The listing builds one solid part. Answer for the finished solid, in the listing's coordinates (mm). A direction names the side the tool comes from. Round coordinates to 2 decimals unless told otherwise and drop trailing zeros. Loops run counter-clockwise (first coordinate to the right, second up) from the corner with the lowest first, then second, coordinate; pieces in that order, holes last. Notation, with made-up numbers: (79, 3.25) - (85, 3.25) arc R17 cw to (85, 35.25) - close; hole circle Ø11 at (-14, -18.5). An arc over 180 degrees is marked (long way). Write item = value, one per line. Start each with the question number.
1) Straight lines are drawn through the part: line 1 along Y through (x, z) = (29, 17.5); line 2 along X through (y, z) = (10.5, 11); line 3 along X through (y, z) = (4.25, 4.25). For each, find the intervals that lie inside material, in ascending order.
2) Section B-B, the plane z = 11 is taken. Determine the outline of the cut face in (x, y), and give its area (3 significant figures).
3) Section C-C, the plane x = 29 is taken. Determine the outline of the cut face in (y, z), and give its area (3 significant figures).
4) Section A-A, the plane y = 6 is taken. Determine the outline of the cut face in (x, z), and give its area (3 significant figures).
5) A tool of negligible diameter and unlimited length cuts with its end or side. For faces 4 (the flat face through (33, 15, 9)), 5 (the flat face through (1, 15, 9)), 6 (the cylindrical face through (3, 24, 13)), 7 (the flat face through (17, 15, 21.5)), from which of +Z, -Z, +X, -X, +Y, -Y can it reach the whole face along a straight path? Write none if from no direction.
6) For a pull along Z with two mould halves and no side action, classify faces 1 (the flat face through (14, 2, 8)), 2 (the flat face through (5, 15, 22)), 3 (the flat face through (29, 15, 4)) as released by +Z, released by -Z, zero draft, split by the parting line, or undercut.
7) Section D-D, the plane y = 3 is taken. Determine the outline of the cut face in (x, z).
8) Given pin 1 Ø4 at (x, y) = (28.5, 19) entering from -Z; pin 2 Ø5 at (y, z) = (13, 7.5) entering from -X; pin 3 Ø2 at (x, z) = (11.5, 12) entering from +Y; pin 4 Ø5 at (x, z) = (17, 11) entering from -Y, each flat-ended and moving along its own axis, determine where each tip first touches the part or whether it passes through.
from build123d import *

# Parameters (mm, degrees)
CYLINDER002_R          = 7.5
CYLINDER002_DEPTH      = 4
CYLINDER002_ROLL_ANGLE = 90
BOX003_W               = 7
BOX003_H               = 34
BOX003_DEPTH           = 0.5
PAD001_DEPTH           = 27
BOX002_W               = 8
BOX002_H               = 22
BOX002_DEPTH           = 4
BOX001_W               = 1
BOX001_H               = 19
BOX001_DEPTH           = 14
PAD_DEPTH              = 31
CYLINDER001_R          = 2
CYLINDER001_DEPTH      = 30
CYLINDER_R             = 4
CYLINDER_DEPTH         = 40
CYLINDER_ROLL_ANGLE    = 90
BOX_W                  = 17
BOX_H                  = 15
BOX_DEPTH              = 22


with BuildPart() as cilindro002:
    # Cylinder002 → Cylinder002 (new body)
    with BuildSketch(Plane.XY):
        Circle(CYLINDER002_R)
    extrude(amount=CYLINDER002_DEPTH)


with BuildPart() as cilindro002_1:
    # Cylinder002 roll: moved
    add(cilindro002.part.rotate(Axis((0, 0, 0), (1, 0, 0)), CYLINDER002_ROLL_ANGLE))


with BuildPart() as cilindro002_2:
    # Cylinder002 placement: moved
    add(cilindro002_1.part.moved(Location((17, 2, 11))))


with BuildPart() as cubo003:
    # Box003 → Box003 (new body)
    with BuildSketch(Plane(origin=(10, 0, 21.5), x_dir=(1, 0, 0), z_dir=(0, 0, 1))):
        with Locations((3.5, 17)):
            Rectangle(BOX003_W, BOX003_H)
    extrude(amount=BOX003_DEPTH)


with BuildPart() as body001:
    # Sketch001 → Pad001 (new body)
    with BuildSketch(Plane.XZ):
        Polygon((0, 0), (4, 0), (0, 4), align=None)
    extrude(amount=PAD001_DEPTH)


with BuildPart() as body001_1:
    # Body001 placement: moved
    add(body001.part.moved(Location((9, 20, 0))))


with BuildPart() as cubo002:
    # Box002 → Box002 (new body)
    with BuildSketch(Plane(origin=(1, 0, 0), x_dir=(1, 0, 0), z_dir=(0, 0, 1))):
        with Locations((4, 11)):
            Rectangle(BOX002_W, BOX002_H)
    extrude(amount=BOX002_DEPTH)


with BuildPart() as cubo001:
    # Box001 → Box001 (new body)
    with BuildSketch(Plane.XY):
        with Locations((0.5, 9.5)):
            Rectangle(BOX001_W, BOX001_H)
    extrude(amount=BOX001_DEPTH)


with BuildPart() as body:
    # Sketch → Pad (new body)
    with BuildSketch(Plane.XZ):
        Polygon((0, 0), (-1, -8e-06), (-1, 1.999992), align=None)
    extrude(amount=PAD_DEPTH)


with BuildPart() as body_1:
    # Body placement: moved
    add(body.part.moved(Location((1, 18, 14))))


with BuildPart() as cilindro001:
    # Cylinder001 → Cylinder001 (new body)
    with BuildSketch(Plane(origin=(5, 6, -3), x_dir=(1, 0, 0), z_dir=(0, 0, 1))):
        Circle(CYLINDER001_R)
    extrude(amount=CYLINDER001_DEPTH)


with BuildPart() as cilindro:
    # Cylinder → Cylinder (new body)
    with BuildSketch(Plane.XY):
        Circle(CYLINDER_R)
    extrude(amount=CYLINDER_DEPTH)


with BuildPart() as cilindro_1:
    # Cylinder roll: moved
    add(cilindro.part.rotate(Axis((0, 0, 0), (1, 0, 0)), CYLINDER_ROLL_ANGLE))


with BuildPart() as cilindro_2:
    # Cylinder placement: moved
    add(cilindro_1.part.moved(Location((17, 35, 11))))


with BuildPart() as cut007:
    # Box → Box (new body)
    with BuildSketch(Plane.XY):
        with Locations((8.5, 7.5)):
            Rectangle(BOX_W, BOX_H)
    extrude(amount=BOX_DEPTH)

    # Cut: cut Cilindro
    add(cilindro_2.part, mode=Mode.SUBTRACT)

    # Cut001: cut Cilindro001
    add(cilindro001.part, mode=Mode.SUBTRACT)

    # Cut002: cut Body
    add(body_1.part, mode=Mode.SUBTRACT)

    # Cut003: cut Cubo001
    add(cubo001.part, mode=Mode.SUBTRACT)

    # Cut004: cut Cubo002
    add(cubo002.part, mode=Mode.SUBTRACT)

    # Cut005: cut Body001
    add(body001_1.part, mode=Mode.SUBTRACT)

    # Cut006: cut Cubo003
    add(cubo003.part, mode=Mode.SUBTRACT)

    # Cut007: cut Cilindro002
    add(cilindro002_2.part, mode=Mode.SUBTRACT)


with BuildPart() as fusion:
    # mirror: instance of Cut007
    add(cut007.part.mirror(Plane(origin=(17, 0, 0.020863), x_dir=(0, -1, 0), z_dir=(1, 0, 0))))

    # Fusion: union Cut007
    add(cut007.part)


with BuildPart() as mirror_of_fusion:
    # mirror001: instance of Fusion
    add(fusion.part.mirror(Plane(origin=(34, 15, 22), x_dir=(1, 0, 0), z_dir=(0, 1, 0))))


with BuildPart() as fusion001:
    # Fusion001 base: copy of Fusion
    add(fusion.part)

    # Fusion001: union Mirror of Fusion
    add(mirror_of_fusion.part)


solid = fusion001.part
Geometry check:
q1.line_1 = 0 to 4, 8 to 22, 26 to 30
q1.line_2 = 1 to 13, 21 to 33
q1.line_3 = 1 to 4.03, 5.97 to 28.03, 29.97 to 33
q2.outline = (1, 0) - (9.5, 0) - (9.5, 2) - (13, 2) - (13, 28) - (9.5, 28) - (9.5, 30) - (1, 30) - close; (21, 2) - (24.5, 2) - (24.5, 0) - (33, 0) - (33, 30) - (24.5, 30) - (24.5, 28) - (21, 28) - close; hole circle Ø4 at (5, 6); hole circle Ø4 at (5, 24); hole circle Ø4 at (29, 6); hole circle Ø4 at (29, 24)
q2.area = 642 mm2
q3.outline = (0, 4) - (4, 4) - (4, 22) - (0, 22) - close; (8, 4) - (22, 4) - (22, 22) - (8, 22) - close; (26, 4) - (30, 4) - (30, 22) - (26, 22) - close
q3.area = 396 mm2
q4.outline = (0, 16) - (1, 14) - (1, 4) - (3, 4) - (3, 22) - (0, 22) - close; (7, 4) - (9, 4) - (13, 0) - (21, 0) - (25, 4) - (27, 4) - (27, 22) - (24, 22) - (24, 21.5) - (10, 21.5) - (10, 22) - (7, 22) - close; (31, 4) - (33, 4) - (33, 14) - (34, 16) - (34, 22) - (31, 22) - close; hole circle Ø8 at (17, 11)
q4.area = 437 mm2
q5.face_4 = -Z, +X, +Y, -Y
q5.face_5 = -Z, -X, +Y, -Y
q5.face_6 = +Z, -Z
q5.face_7 = +Z, +Y, -Y
q6.face_1 = undercut
q6.face_2 = released by +Z
q6.face_3 = released by -Z
q7.outline = (0, 16) - (1, 14) - (1, 4) - (9, 4) - (13, 0) - (21, 0) - (25, 4) - (33, 4) - (33, 14) - (34, 16) - (34, 22) - (24, 22) - (24, 21.5) - (10, 21.5) - (10, 22) - (0, 22) - close; hole circle Ø8 at (17, 11)
q8.pin_1 = 4
q8.pin_2 = 1
q8.pin_3 = 28
q8.pin_4 = through
